Job drawing, mm, ordinate dimensions from the low corner. One solid piece. A direction names the side the tool comes from. Coordinates: 2 decimals unless noted, no trailing zeros. Loops run counter-clockwise (first coordinate to the right, second up) from the corner with the lowest first, then second, coordinate; pieces in that order, holes last. Notation, with made-up numbers: M 46.5,12 L 61.5,12 A19 cw 61.5,42 Z; hole C -17,-20.75 d1. An arc over 180 degrees is marked long. Answer as a JSON object with one key per item and string values. Group by question number.
1. Saw through at D-D on y = 21. Count the separate pieces of the cut face and the enclosed holes in it, then the cut area to 3 significant figures.
2. Saw through at A-A on x = 20.5. Write the cut outline in (y, z), then the cut area to 3 significant figures.
3. 3-axis set-ups, long thin cutter, end or side, ignore diameter. For the marked faces 1 and 2: which of +Z, -Z, +X, -X, +Y, -Y reach the whole face in a straight line?
4. Saw through at B-B on z = 5.5. Write the cut outline in (x, y), then the cut area to 3 significant figures.
5. Drop a flat-ended pin along its axis: pin 1 Ø2.5 at (x, z) = (56.5, 12.5) entering from +Y. Give the stop position or say it passes through.
6. Drill centre lines: L1, parallel to Z at x = 19.5, y = 11; L2, parallel to X at y = 0.8, z = 5.5; L3, parallel to Y at x = 63.5, z = 1.65. Where is each one in solid material? Low to high.
7. Saw through at C-C on y = 4.25. Write the cut outline in (x, z).
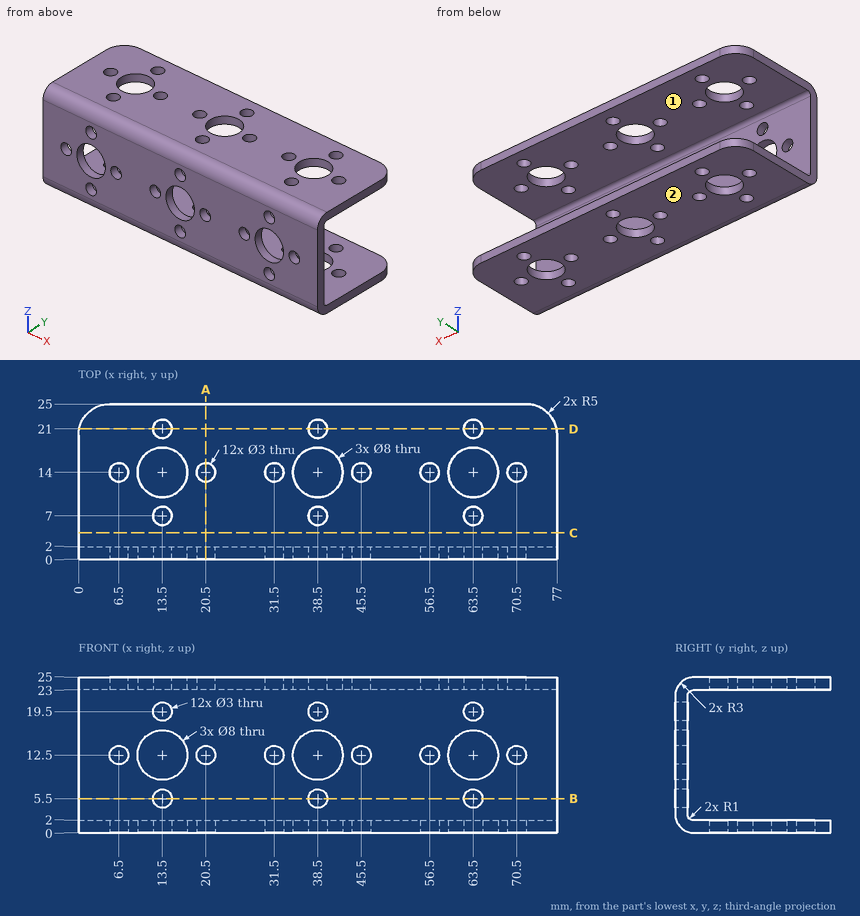
Outcome:
{
 "1": {"separate pieces": "8", "enclosed holes": "0", "area": "271 mm²"},
 "2": {"outline": "M 0,3 A3 ccw 3,0 L 12.5,0 L 12.5,2 L 3,2 A1 cw 2,3 L 2,11 L 0,11 Z; M 0,14 L 2,14 L 2,22 A1 cw 3,23 L 12.5,23 L 12.5,25 L 3,25 A3 ccw 0,22 Z; M 15.5,0 L 25,0 L 25,2 L 15.5,2 Z; M 15.5,23 L 25,23 L 25,25 L 15.5,25 Z", "area": "121 mm²"},
 "3": {"face 1": "+X, -X, +Y", "face 2": "-Z, +X, -X, +Y, -Y"},
 "4": {"outline": "M 0,0 L 12,0 L 12,2 L 0,2 Z; M 15,0 L 37,0 L 37,2 L 15,2 Z; M 40,0 L 62,0 L 62,2 L 40,2 Z; M 65,0 L 77,0 L 77,2 L 65,2 Z", "area": "136 mm²"},
 "5": {"pin 1": "passes through"},
 "6": {"L1": "z = 0 to 2, 23 to 25", "L2": "x = 0 to 12, 15 to 37, 40 to 62, 65 to 77", "L3": "y = 0.32 to 5.5, 8.5 to 10, 18 to 19.5, 22.5 to 25"},
 "7": {"outline": "M 0,0 L 77,0 L 77,2 L 0,2 Z; M 0,23 L 77,23 L 77,25 L 0,25 Z"}
}
